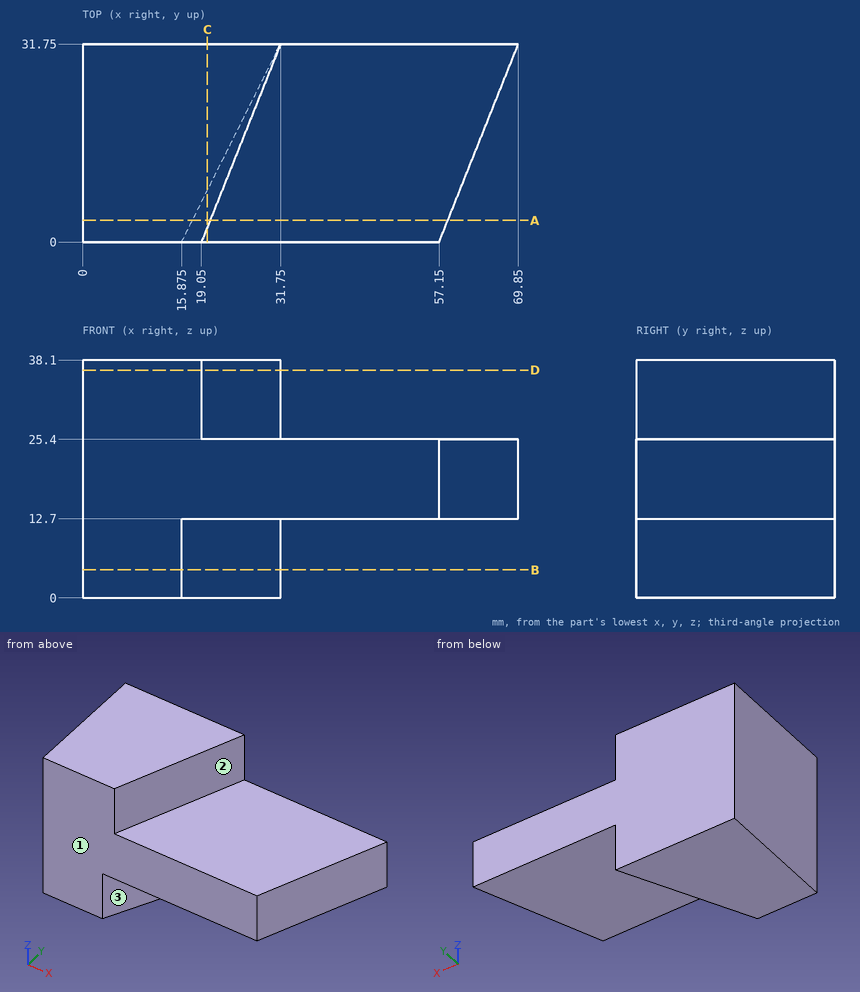
Job drawing, mm, ordinate dimensions from the low corner. One solid piece. A direction names the side the tool comes from. Give positions to 0.01 mm unless a question says otherwise; leave off trailing zeros. Loops run counter-clockwise (first coordinate to the right, second up) from the corner with the lowest first, then second, coordinate; pieces in that order, holes last. Notation, with made-up numbers: (-34.5, 61) -> (6.5, 61) arc R9 cw to (6.5, 66) -> close; hole circle Ø7 at (31.25, -29.5). An arc over 180 degrees is marked (long way). Use a Markdown table: item, result. Add a question column.
(1) Slice it at D-D on z = 36.5. List the corners of the cut face in (x, y).
(2) Slice it at C-C on x = 20. List the corners of the cut face in (y, z) (3 decimals), and give its area (3 significant figures).
(3) Drop flat-ended pins along their axis: pin 1 Ø9.5 at (x, y) = (35, 20) entering from -Z; pin 2 Ø9.5 at (x, y) = (42, 15) entering from +Z. Give the stop position or say it passes through.
(4) Slice it at B-B on z = 4.5. List the corners of the cut face in (x, y) (3 decimals).
(5) Tool access for the marked faces 1, 2 and 3: list every direction of +Z, -Z, +X, -X, +Y, -Y with a clear straight run to the whole face (end or side of a thin tool).
(6) Wall check: line 1 along Z through (x, y) = (42, 1.5); line 2 along X through (y, z) = (30, 27); line 3 along X through (y, z) = (28, 30). Give the ranges that are in metal, low to high.
(7) Slice it at A-A on y = 3.5. List the corners of the cut face in (x, z) (3 decimals).
Filled sheet:
| question | item | result |
|---|---|---|
| 1 | outline | (0, 0) -> (19.05, 0) -> (31.75, 31.75) -> (0, 31.75) -> close |
| 2 | outline | (0, 12.7) -> (8.25, 12.7) -> (8.25, 0) -> (31.75, 0) -> (31.75, 38.1) -> (2.375, 38.1) -> (2.375, 25.4) -> (0, 25.4) -> close |
| 2 | area | 1,070 mm2 |
| 3 | pin 1 | z = 12.7 |
| 3 | pin 2 | z = 25.4 |
| 4 | outline | (0, 0) -> (15.875, 0) -> (31.75, 31.75) -> (0, 31.75) -> close |
| 5 | face 1 | +Z, -Z, +X, -X, -Y |
| 5 | face 2 | +Z, +X, -Y |
| 5 | face 3 | -Z, +X, -Y |
| 6 | line 1 | 12.7 to 25.4 |
| 6 | line 2 | 0 to 31.05 |
| 6 | line 3 | 0 to 30.25 |
| 7 | outline | (0, 0) -> (17.625, 0) -> (17.625, 12.7) -> (58.55, 12.7) -> (58.55, 25.4) -> (20.45, 25.4) -> (20.45, 38.1) -> (0, 38.1) -> close |
